Design review of the part built by this model. Coordinates are the model's own, in mm. Face numbers are marked on the shaded views. A direction names the side the tool comes from. Round coordinates to 2 decimals unless told otherwise and drop trailing zeros. Write each loop counter-clockwise with the first axis right and the second up, starting at its lowest first coordinate (ties: lowest second). Pieces come first, ordered by that corner, then holes. Notation, with made-up numbers: (50.25, -9.5) -> (70.25, -9.5) arc R28 cw to (70.25, 17.5) -> close; hole circle Ø4 at (-34.75, 57.25). An arc over 180 degrees is marked (long way). One line per question, with ' | ' between items. Start each with the question number.
1) Consider section A-A (z = 17.25). Give the boundary of the cut face in (x, y).
2) For the marked faces 1, 2 and 3, list the 3-axis set-ups (+Z, -Z, +X, -X, +Y, -Y) from which the entire face can be reached by the end or side of a thin tool; tool diameter is ignored.
3) Consider section D-D (y = -5). Give the boundary of the cut face in (x, z).
4) Consider section C-C (y = 0). Give the boundary of the cut face in (x, z), then the cut area to 3 significant figures.
5) For probe 1 along Y at (x, z) = (16.5, 5) (3 decimals); probe 2 along Y at (x, z) = (37.5, 8) (3 decimals); probe 3 along X at (y, z) = (0.5, 11.5), list the stretches that pass through material, from the lowest coordinate up.
6) Consider section B-B (x = 27.5). Give the boundary of the cut face in (y, z) (3 decimals).
7) Insertion check: pin 1 Ø3 at (y, z) = (5.5, 9) entering from +X; pin 2 Ø1.5 at (x, z) = (38, 7.5) entering from +Y; pin 3 Ø8 at (y, z) = (6, 4) entering from -X. Each pin has a flat end and moves straight along its axis. Give the tip position at first contact, or say it passes through.
8) Mouldability with a two-part tool opening along X and no side actions: class the marked faces 4, 5 and 6 as +X half, -X half, draft (parallel to the pull), parting line (faces both ways), or undercut.
```python
from build123d import *

# Parameters (mm, degrees)
BOSS_EXTRUDE1_DEPTH = 20
FILLET1_R           = 10
FILLET2_R           = 1


with BuildPart() as part:
    # Sketch1 → Boss-Extrude1 (new body)
    with BuildSketch(Plane.XY):
        with BuildLine():
            Line((50, 10), (50, 8.75))
            Line((50, 8.75), (44.792027113, 7.760398644))
            Line((44.792027113, 7.760398644), (0, 10))
            ThreePointArc((0, 10), (-10, 0), (0, -10))
            Line((0, -10), (44.792027113, -7.760398644))
            Line((44.792027113, -7.760398644), (50, -8.75))
            Line((50, -8.75), (50, -10))
            Line((50, -10), (0, -12.5))
            ThreePointArc((0, -12.5), (-12.5, 0), (0, 12.5))
            Line((0, 12.5), (50, 10))
        make_face()
    extrude(amount=BOSS_EXTRUDE1_DEPTH)

    # Fillet1
    fillet1_edges = [part.edges().sort_by_distance(p)[0] for p in [
        (44.792027113, 7.760398644, 10),
        (44.792027113, -7.760398644, 10),
    ]]
    fillet(fillet1_edges, radius=FILLET1_R)

    # Fillet2
    fillet2_edges = [part.edges().sort_by_distance(p)[0] for p in [
        (50, -8.75, 10),
        (50, 8.75, 10),
    ]]
    fillet(fillet2_edges, radius=FILLET2_R)


solid = part.part
```
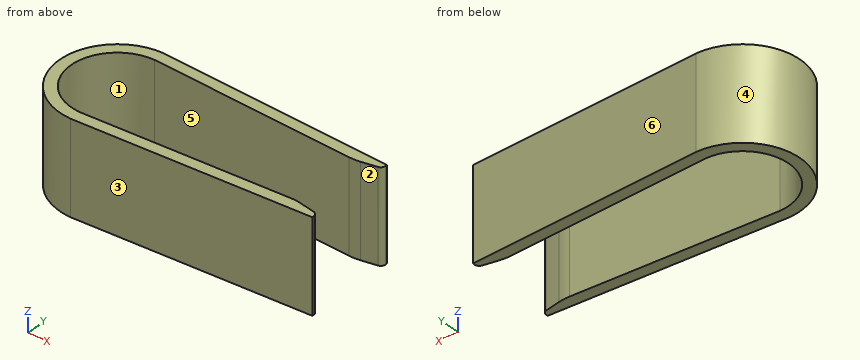
From the geometry:
1) outline: (0, -12.5) -> (50, -10) -> (50, -9.58) arc R1 ccw to (49.19, -8.6) -> (45.97, -7.98) arc R10 ccw to (43.6, -7.82) -> (0, -10) arc R10 cw to (0, 10) -> (43.6, 7.82) arc R10 ccw to (45.97, 7.98) -> (49.19, 8.6) arc R1 ccw to (50, 9.58) -> (50, 10) -> (0, 12.5) arc R12.5 ccw to start
2) face 1: +Z, -Z | face 2: +Z, -Z, +X | face 3: +Z, -Z, +X, -Y
3) outline: (-11.46, 0) -> (-8.66, 0) -> (-8.66, 20) -> (-11.46, 20) -> close
4) outline: (-12.5, 0) -> (-10, 0) -> (-10, 20) -> (-12.5, 20) -> close | area: 50.0 mm2
5) probe 1: y = -11.675 to -9.175, 9.175 to 11.675 | probe 2: y = -10.625 to -8.125, 8.125 to 10.625 | probe 3: x = -12.49 to -9.99
6) outline: (-11.125, 0) -> (-8.625, 0) -> (-8.625, 20) -> (-11.125, 20) -> close; (8.625, 0) -> (11.125, 0) -> (11.125, 20) -> (8.625, 20) -> close
7) pin 1: stops at x = -7.14 | pin 2: stops at y = 10.64 | pin 3: stops at x = -12.34
8) face 4: -X half | face 5: undercut | face 6: +X half
